from build123d import *

# Parameters (mm, degrees)
SKETCH1_R           = 8.5
SKETCH1_R_2         = 4.765
BOSS_EXTRUDE1_DEPTH = 8
SKETCH2_R           = 5.5
CUT_EXTRUDE1_DEPTH  = 36.397740041
SKETCH7_W           = 11
SKETCH7_H           = 10
CUT_EXTRUDE3_DEPTH  = 16
SKETCH14_R          = 1.585
CUT_EXTRUDE5_DEPTH  = 22
SKETCH15_W          = 11
SKETCH15_H          = 10
CUT_EXTRUDE6_DEPTH  = 22


with BuildPart() as part:
    # Sketch1 → Boss-Extrude1 (new, symmetric)
    # profile 1 of 3: a face of its own
    with BuildSketch(Plane.XY):
        with BuildLine():
            Line((-22, 0), (-8.141153884, -2.443688492))
            ThreePointArc((-8.141153884, -2.443688492), (-6.819873612, 5.073393727), (0, 8.5))
            Line((0, 8.5), (-22, 8.5))
            Line((-22, 8.5), (-22, 0))
        make_face()
    # profile 2 of 3: a face of its own
    with BuildSketch(Plane.XY):
        Circle(SKETCH1_R)
        Circle(SKETCH1_R_2, mode=Mode.SUBTRACT)
    # profile 3 of 3: a face of its own
    with BuildSketch(Plane.XY):
        with BuildLine():
            ThreePointArc((8.5, 0), (6.01040764, -6.01040764), (0, -8.5))
            Line((0, -8.5), (30, -8.5))
            Line((30, -8.5), (30, 0))
            Line((30, 0), (8.5, 0))
        make_face()
    extrude(amount=BOSS_EXTRUDE1_DEPTH, both=True)

    # Sketch2 → Cut-Extrude1 (cut, through all)
    with BuildSketch(Plane(origin=(0, 8.5, 0), x_dir=(1, 0, 0), z_dir=(0, 1, 0))):
        with Locations(Location((0, 0, 0), (0, 0, 270))):
            Circle(SKETCH2_R)
    extrude(amount=-CUT_EXTRUDE1_DEPTH, mode=Mode.SUBTRACT)

    # Sketch7 → Cut-Extrude3 (cut)
    with BuildSketch(Plane(origin=(0, 8.5, 0), x_dir=(1, 0, 0), z_dir=(0, 1, 0))):
        with Locations((-16.5, 0)):
            Rectangle(SKETCH7_W, SKETCH7_H)
    extrude(amount=-CUT_EXTRUDE3_DEPTH, mode=Mode.SUBTRACT)

    # Sketch13 → Cut-Loft6 section 0
    with BuildSketch(Plane(origin=(0, 8.5, 0), x_dir=(1, 0, 0), z_dir=(0, 1, 0))):
        with BuildLine():
            Line((-22, -6.5), (-22, -8))
            Line((-22, -8), (-11.095577143, -8))
            Line((-11.095577143, -8), (-22, -6.5))
        make_face()
    # Sketch12 → Cut-Loft6 section 1
    with BuildSketch(Plane(origin=(-0.663381171, -3.762221577, 0), x_dir=(0.9848077530122088, -0.17364817766692656, 0), z_dir=(-0.17364817766692653, -0.9848077530122087, 0))):
        with BuildLine():
            Line((-10.59312941, 8), (-21.665770566, 6.5))
            Line((-21.665770566, 6.5), (-21.665770566, 8))
            Line((-21.665770566, 8), (-10.59312941, 8))
        make_face()
    cut_loft6 = loft(mode=Mode.SUBTRACT)

    # Mirror1: Cut-Loft6 across plane
    add(cut_loft6.mirror(Plane.XY), mode=Mode.SUBTRACT)

    # Sketch14 → Cut-Extrude5 (cut, symmetric)
    with BuildSketch(Plane.XY):
        with Locations(Location((-19.5, 4.25, 0), (0, 0, 180))):
            Circle(SKETCH14_R)
        with Locations((27.5, -4.25)):
            Circle(SKETCH14_R)
    extrude(amount=CUT_EXTRUDE5_DEPTH, both=True, mode=Mode.SUBTRACT)

    # Sketch15 → Cut-Extrude6 (cut, symmetric)
    with BuildSketch(Plane(origin=(0, 0, 0), x_dir=(1, 0, 0), z_dir=(0, 1, 0))):
        Polygon((30, 8), (19, 8), (30, 6.5), align=None)
        with Locations((24.5, 0)):
            Rectangle(SKETCH15_W, SKETCH15_H)
        Polygon((30, -6.5), (19, -8), (30, -8), align=None)
    extrude(amount=CUT_EXTRUDE6_DEPTH, both=True, mode=Mode.SUBTRACT)


solid = part.part
Geometry: final body of the model. Coordinates: model frame, mm. A direction names the side the tool comes from. Give positions to 0.01 mm unless a question says otherwise; leave off trailing zeros. Order: outer loops, then holes, each group sorted by start corner. A loop starts at its lowest first (then second) coordinate and runs counter-clockwise, first axis right, second up. Notation, with made-up numbers: (8.5, -10) -> (35.5, -10) arc R18 ccw to (35.5, 12) -> close; hole circle Ø8 at (48.25, 18). An arc over 180 degrees is marked (long way). Put each result on its own line as item: value.
Q1. Section B-B, the plane x = 1.5. Return loops of the section in (y, z), then the cut area to 3 significant figures.
Here are the results:
outline: (-8.5, -8) -> (-4.52, -8) -> (-4.52, -5.29) -> (-8.5, -5.29) -> close; (-8.5, 5.29) -> (-4.52, 5.29) -> (-4.52, 8) -> (-8.5, 8) -> close; (4.52, -8) -> (8.37, -8) -> (8.37, -5.29) -> (4.52, -5.29) -> close; (4.52, 5.29) -> (8.37, 5.29) -> (8.37, 8) -> (4.52, 8) -> close
area: 42.4 mm^2
Q2. Reachability of faces 5 (the face through (-17, 3, 5)), 6 (the face through (15, -8.5, 0)), 7 (the face through (24, -4, -5)), 8 (the face through (24.42, -4.31, -7.26)), 9 (the face through (17, 0, 0)) from +Z, -Z, +X, -X, +Y, -Y: full face, straight path, thin tool, end or side. Return the list, or none.
Here are the results:
face 5: -X, +Y, -Y
face 6: +Z, -Z, +X, -X, -Y
face 7: +X, +Y, -Y
face 8: -Z, +X, +Y, -Y
face 9: +Z, -Z, +X, +Y
Q3. Material intervals for L1, parallel to X at y = 4.25, z = -5.5 (3 decimals); L2, parallel to Y at x = 27.5, z = -6.35 (3 decimals); L3, parallel to Y at x = 0, z = -6.35 (3 decimals), sorted ascending.
Here are the results:
L1: x = -22 to -21.085, -17.915 to -2.155, 2.155 to 7.361
L2: y = -8.5 to -5.835, -2.665 to 0
L3: y = -8.5 to -4.765, 4.765 to 8.5
Q4. Section A-A, the plane z = -2. Return loops of the section in (x, y).
Here are the results:
outline: (-11, -1.94) -> (-8.14, -2.44) arc R8.5 ccw to (-5.12, -6.78) -> (-5.12, 8.5) -> (-11, 8.5) -> close; (5.12, -8.5) -> (19, -8.5) -> (19, 0) -> (8.5, 0) arc R8.5 ccw to (5.12, 6.78) -> close
Q5. Draft query along X for faces 1 (the face through (-17, 3, -5)), 2 (the face through (19, -4, 0)), 3 (the face through (25.917, -4.18, -6.024)), 4 (the face through (-5.37, 0.12, -1.19)). Return one class per face: released by +X, released by -X, zero draft, split by the parting line, or undercut.
Here are the results:
face 1: zero draft
face 2: released by +X
face 3: undercut
face 4: undercut
Q6. Pin query (flat end, axial travel): pin 1 (5 mm diameter, centred on x = 27.5, y = -4.25, fed in from +Z); pin 2 (4 mm diameter, centred on y = -6, z = -1.5, fed in from +X); pin 3 (5 mm diameter, centred on x = -16.5, y = 4.5, fed in from +Z). Return the tip coordinate at first contact, or that it passes through.
Here are the results:
pin 1: stops at z = 7.18
pin 2: stops at x = 19
pin 3: stops at z = 7.6
Q7. Section C-C, the plane y = -3.5. Return loops of the section in (x, z).
Here are the results:
outline: (-7.75, -8) -> (-3.23, -8) -> (-3.23, -4.45) arc R5.5 cw to (-3.23, 4.45) -> (-3.23, 8) -> (-7.75, 8) -> close; (3.23, -8) -> (19, -8) -> (26.1, -7.03) -> (26.1, -5) -> (19, -5) -> (19, 5) -> (26.1, 5) -> (26.1, 7.03) -> (19, 8) -> (3.23, 8) -> (3.23, 4.45) arc R5.5 cw to (3.23, -4.45) -> close; (28.9, -6.65) -> (30, -6.5) -> (30, -5) -> (28.9, -5) -> close; (28.9, 5) -> (30, 5) -> (30, 6.5) -> (28.9, 6.65) -> close
Q8. Section D-D, the plane x = 27.5. Return loops of the section in (y, z) (3 decimals), then the cut area to 3 significant figures.
Here are the results:
outline: (-8.5, -6.841) -> (-5.835, -6.841) -> (-5.835, -5) -> (-8.5, -5) -> close; (-8.5, 5) -> (-5.835, 5) -> (-5.835, 6.841) -> (-8.5, 6.841) -> close; (-2.665, -6.841) -> (0, -6.841) -> (0, -5) -> (-2.665, -5) -> close; (-2.665, 5) -> (0, 5) -> (0, 6.841) -> (-2.665, 6.841) -> close
area: 19.6 mm^2
